Design review of the part built by this model. Coordinates are the model's own, in mm. Coordinates: 2 decimals unless noted, no trailing zeros. Write each loop counter-clockwise with the first axis right and the second up, starting at its lowest first coordinate (ties: lowest second). Pieces come first, ordered by that corner, then holes. Notation, with made-up numbers: M -28.75,44.25 L 8.25,44.25 A15 cw 8.25,48.25 Z; hole C 86,41.25 d10. An arc over 180 degrees is marked long. Write item = value, one per line.
```python
from build123d import *

# Parameters (mm, degrees)
SKETCH1_W           = 10
SKETCH1_H           = 10
SKETCH1_W_2         = 8
SKETCH1_H_2         = 8
BOSS_EXTRUDE1_DEPTH = 300
SKETCH2_R           = 2.05
CUT_EXTRUDE1_DEPTH  = 301.208261046
SKETCH3_R           = 2.05
CUT_EXTRUDE2_DEPTH  = 301.208261046


with BuildPart() as part:
    # Sketch1 → Boss-Extrude1 (new body)
    with BuildSketch(Plane(origin=(0, 0, 0), x_dir=(1, 0, 0), z_dir=(0, 1, 0))):
        Rectangle(SKETCH1_W, SKETCH1_H)
        Rectangle(SKETCH1_W_2, SKETCH1_H_2, mode=Mode.SUBTRACT)
    extrude(amount=BOSS_EXTRUDE1_DEPTH)

    # Sketch2 → Cut-Extrude1 (cut, through all)
    with BuildSketch(Plane(origin=(5, 0, 0), x_dir=(0, 0, -1), z_dir=(1, 0, 0))):
        with Locations((0, 294)):
            Circle(SKETCH2_R)
        with Locations((0, 6)):
            Circle(SKETCH2_R)
    extrude(amount=-CUT_EXTRUDE1_DEPTH, mode=Mode.SUBTRACT)

    # Sketch3 → Cut-Extrude2 (cut, through all)
    with BuildSketch(Plane.XY.offset(5)):
        with Locations((0, 150)):
            Circle(SKETCH3_R)
        with Locations((0, 158)):
            Circle(SKETCH3_R)
        with Locations((0, 166)):
            Circle(SKETCH3_R)
        with Locations((0, 142)):
            Circle(SKETCH3_R)
        with Locations((0, 134)):
            Circle(SKETCH3_R)
    extrude(amount=-CUT_EXTRUDE2_DEPTH, mode=Mode.SUBTRACT)


solid = part.part
```
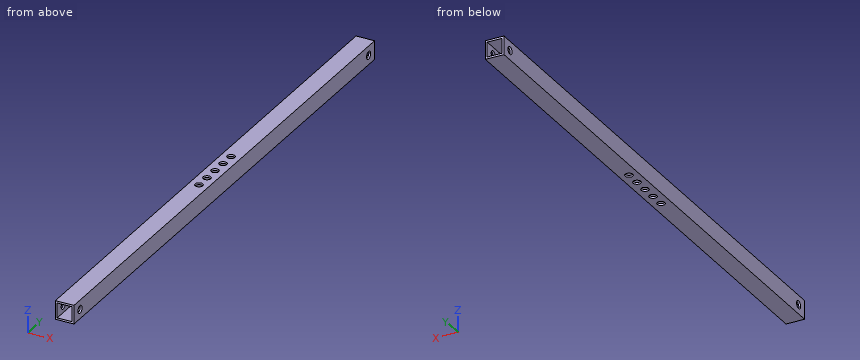
Q1. Wall thickness on line 1 (Y direction, x = 0, z = -4.65); line 2 (Y direction, x = 4.4, z = 0); line 3 (Z direction, x = -2.25, y = 128.5): over which ranges is each line inside the solid? List them lowest first.
Check result:
line_1 = 0 to 131.95, 136.05 to 139.95, 144.05 to 147.95, 152.05 to 155.95, 160.05 to 163.95, 168.05 to 300
line_2 = 0 to 3.95, 8.05 to 291.95, 296.05 to 300
line_3 = -5 to -4, 4 to 5
Q2. Consider section A-A, the plane y = 90. State the section outline as (x, z) points, and give its area (3 significant figures).
Check result:
outline = M -5,-5 L 5,-5 L 5,5 L -5,5 Z; hole M -4,-4 L 4,-4 L 4,4 L -4,4 Z
area = 36.0 mm²
Q3. Consider section C-C, the plane x = -0.5. State how many separate pieces and enclosed holes the cut face has, and give its area (3 significant figures).
Check result:
separate_pieces = 12
enclosed_holes = 0
area = 560 mm²
Q4. Consider section B-B, the plane z = 0. State the section outline as (x, y) points.
Check result:
outline = M -5,0 L -4,0 L -4,3.95 L -5,3.95 Z; M -5,8.05 L -4,8.05 L -4,291.95 L -5,291.95 Z; M -5,296.05 L -4,296.05 L -4,300 L -5,300 Z; M 4,0 L 5,0 L 5,3.95 L 4,3.95 Z; M 4,8.05 L 5,8.05 L 5,291.95 L 4,291.95 Z; M 4,296.05 L 5,296.05 L 5,300 L 4,300 Z
